from build123d import *

# Parameters (mm, degrees)
SKETCH_R   = 2.55
SKETCH_R_2 = 3.6
PAD_DEPTH  = 3


with BuildPart() as part:
    # Sketch → Pad (new body)
    with BuildSketch(Plane.XY):
        with BuildLine():
            ThreePointArc((-29.75, 32.75), (-31.87132, 31.87132), (-32.75, 29.75))
            Line((-32.75, -29.75), (-32.75, 29.75))
            ThreePointArc((-32.75, -29.75), (-31.87132, -31.87132), (-29.75, -32.75))
            Line((29.75, -32.75), (-29.75, -32.75))
            ThreePointArc((29.75, -32.75), (31.87132, -31.87132), (32.75, -29.75))
            Line((32.75, 29.75), (32.75, -29.75))
            ThreePointArc((32.75, 29.75), (31.87132, 31.87132), (29.75, 32.75))
            Line((-29.75, 32.75), (29.75, 32.75))
        make_face()
        Circle(SKETCH_R, mode=Mode.SUBTRACT)
        with Locations((-19.85, -20)):
            Circle(SKETCH_R_2, mode=Mode.SUBTRACT)
        with Locations((19.85, -20)):
            Circle(SKETCH_R_2, mode=Mode.SUBTRACT)
        with Locations((19.85, 20)):
            Circle(SKETCH_R_2, mode=Mode.SUBTRACT)
        with Locations((-19.85, 20)):
            Circle(SKETCH_R_2, mode=Mode.SUBTRACT)
        with BuildLine():
            ThreePointArc((-10, -17.5), (-12.5, -20), (-10, -22.5))
            Line((-10, -22.5), (10, -22.5))
            ThreePointArc((10, -22.5), (12.5, -20), (10, -17.5))
            Line((10, -17.5), (-10, -17.5))
        make_face(mode=Mode.SUBTRACT)
        with BuildLine():
            ThreePointArc((-10, 22.5), (-12.5, 20), (-10, 17.5))
            Line((-10, 17.5), (10, 17.5))
            ThreePointArc((10, 17.5), (12.5, 20), (10, 22.5))
            Line((10, 22.5), (-10, 22.5))
        make_face(mode=Mode.SUBTRACT)
    extrude(amount=PAD_DEPTH)


solid = part.part
CAD build for the part. Positions are in the model's coordinates, mm. A direction names the side the tool comes from. Give positions to 0.01 mm unless a question says otherwise; leave off trailing zeros. Write each loop counter-clockwise with the first axis right and the second up, starting at its lowest first coordinate (ties: lowest second). Pieces come first, ordered by that corner, then holes. Notation, with made-up numbers: (53.5, -28.5) - (78.5, -28.5) arc R20 cw to (78.5, -20.5) - close; hole circle Ø7 at (1, 6.25). An arc over 180 degrees is marked (long way). Answer as CSV lines item,"result".
Q1. Pull direction Y, two halves, no side cores. Call faces 3 (the face through (32.75, 0, 1)), 4 (the face through (-12.5, 20.1, 1.5)), 5 (the face through (31.85, -31.89, 1.48)): released by +Y, released by -Y, zero draft, split by the parting line, or undercut.
Result set:
face 3,"zero draft"
face 4,"undercut"
face 5,"released by -Y"
Q2. Drill centre lines: line 1 (Y direction, x = 0, z = 2.1); line 2 (Y direction, x = -19.85, z = 2); line 3 (Y direction, x = 8, z = 0.55). Where is each one in solid material? Low to high. Write a range as from..to.
Result set:
line 1,"-32.75..-22.5, -17.5..-2.55, 2.55..17.5, 22.5..32.75"
line 2,"-32.75..-23.6, -16.4..16.4, 23.6..32.75"
line 3,"-32.75..-22.5, -17.5..17.5, 22.5..32.75"
Q3. Band-saw the part on D-D (y = -20). Give the cut face in (x, z), and give its area (3 significant figures).
Result set:
outline,"(-32.75, 0) - (-23.45, 0) - (-23.45, 3) - (-32.75, 3) - close; (-16.25, 0) - (-12.5, 0) - (-12.5, 3) - (-16.25, 3) - close; (12.5, 0) - (16.25, 0) - (16.25, 3) - (12.5, 3) - close; (23.45, 0) - (32.75, 0) - (32.75, 3) - (23.45, 3) - close"
area,"78.3 mm²"
Q4. Band-saw the part on C-C (z = 2.05). Give the cut face in (x, y), and give its area (3 significant figures).
Result set:
outline,"(-32.75, -29.75) arc R3 ccw to (-29.75, -32.75) - (29.75, -32.75) arc R3 ccw to (32.75, -29.75) - (32.75, 29.75) arc R3 ccw to (29.75, 32.75) - (-29.75, 32.75) arc R3 ccw to (-32.75, 29.75) - close; hole circle Ø7.2 at (-19.85, -20); hole circle Ø7.2 at (-19.85, 20); hole (-10, -22.5) - (10, -22.5) arc R2.5 ccw to (10, -17.5) - (-10, -17.5) arc R2.5 ccw to start; hole (-10, 17.5) - (10, 17.5) arc R2.5 ccw to (10, 22.5) - (-10, 22.5) arc R2.5 ccw to start; hole circle Ø5.1 at (0, 0); hole circle Ø7.2 at (19.85, -20); hole circle Ø7.2 at (19.85, 20)"
area,"3,860 mm²"
Q5. 3-axis set-ups, long thin cutter, end or side, ignore diameter. For faces 1 (the face through (-32.75, 0, 1)), 2 (the face through (0, 22.5, 1)): which of +Z, -Z, +X, -X, +Y, -Y reach the whole face in a straight line?
Result set:
face 1,"+Z, -Z, -X, +Y, -Y"
face 2,"+Z, -Z"
Q6. Band-saw the part on A-A (x = -19.85). Give the cut face in (y, z), and give its area (3 significant figures).
Result set:
outline,"(-32.75, 0) - (-23.6, 0) - (-23.6, 3) - (-32.75, 3) - close; (-16.4, 0) - (16.4, 0) - (16.4, 3) - (-16.4, 3) - close; (23.6, 0) - (32.75, 0) - (32.75, 3) - (23.6, 3) - close"
area,"153 mm²"
Q7. Band-saw the part on B-B (y = 0). Give the cut face in (x, z), and give its area (3 significant figures).
Result set:
outline,"(-32.75, 0) - (-2.55, 0) - (-2.55, 3) - (-32.75, 3) - close; (2.55, 0) - (32.75, 0) - (32.75, 3) - (2.55, 3) - close"
area,"181 mm²"
